```python
from build123d import *

# Parameters (mm, degrees)
IZIM1_R                     = 10
Y_KSEKLIK_EKSTR_ZYON1_DEPTH = 215
Y_KSEKLIK_EKSTR_ZYON2_DEPTH = 150


with BuildPart() as part:
    # Çizim1 → Yükseklik-Ekstrüzyon1 (new body)
    with BuildSketch(Plane.XY):
        Circle(IZIM1_R)
    extrude(amount=-Y_KSEKLIK_EKSTR_ZYON1_DEPTH)

    # Çizim2 → Yükseklik-Ekstrüzyon2 (add)
    with BuildSketch(Plane.XY.offset(-40)):
        with BuildLine():
            ThreePointArc((-9.797958971, -2), (-10, 0), (-9.797958971, 2))
            Line((-9.797958971, 2), (-11.832159566, 2))
            ThreePointArc((-11.832159566, 2), (-12, 0), (-11.832159566, -2))
            Line((-11.832159566, -2), (-9.797958971, -2))
        make_face()
        with BuildLine():
            Line((-1.1256228, 9.936446715), (-1.754225354, 11.871086446))
            ThreePointArc((-1.754225354, 11.871086446), (-3.708203932, 11.412678196), (-5.558451419, 10.635018469))
            Line((-5.558451419, 10.635018469), (-4.929848865, 8.700378737))
            ThreePointArc((-4.929848865, 8.700378737), (-3.090169944, 9.510565163), (-1.1256228, 9.936446715))
        make_face()
        with BuildLine():
            Line((8.396847665, 8.572802885), (6.751144813, 7.377129775))
            ThreePointArc((6.751144813, 7.377129775), (8.090169944, 5.877852523), (9.102285822, 4.141061797))
            Line((9.102285822, 4.141061797), (10.747988674, 5.336734907))
            ThreePointArc((10.747988674, 5.336734907), (9.708203932, 7.053423028), (8.396847665, 8.572802885))
        make_face()
        with BuildLine():
            Line((10.747988674, -5.336734907), (9.102285822, -4.141061797))
            ThreePointArc((9.102285822, -4.141061797), (8.090169944, -5.877852523), (6.751144813, -7.377129775))
            Line((6.751144813, -7.377129775), (8.396847665, -8.572802885))
            ThreePointArc((8.396847665, -8.572802885), (9.708203932, -7.053423028), (10.747988674, -5.336734907))
        make_face()
        with BuildLine():
            ThreePointArc((-1.1256228, -9.936446715), (-3.090169944, -9.510565163), (-4.929848865, -8.700378737))
            Line((-4.929848865, -8.700378737), (-5.558451419, -10.635018469))
            ThreePointArc((-5.558451419, -10.635018469), (-3.708203932, -11.412678196), (-1.754225354, -11.871086446))
            Line((-1.754225354, -11.871086446), (-1.1256228, -9.936446715))
        make_face()
    extrude(amount=-Y_KSEKLIK_EKSTR_ZYON2_DEPTH)


solid = part.part
```
Model file for the job. Use its own axes, mm. A direction names the side the tool comes from. Round coordinates to 2 decimals unless told otherwise and drop trailing zeros. Loops run counter-clockwise (first coordinate to the right, second up) from the corner with the lowest first, then second, coordinate; pieces in that order, holes last. Notation, with made-up numbers: M -19,16.25 L -10,16.25 A25 ccw -10,50.25 Z; hole C 32,12.5 d2. An arc over 180 degrees is marked long. Put each result on its own line as item: value. Start each with the question number.
Item 1: 3-axis set-ups, long thin cutter, end or side, ignore diameter. For faces 1 (the face through (9, 6, -190)), 2 (the face through (-3.735, -11.404, -113.95)), 3 (the face through (9, 6, -40)), 4 (the face through (9, -6, -190)), 5 (the face through (9, -6, -40)): which of +Z, -Z, +X, -X, +Y, -Y reach the whole face in a straight line?
Item 2: Cut at B-B (z = -91.5). List the corners of the cut face in (x, y), then the cut area to 3 significant figures.
Item 3: Drop flat-ended pins along their axis: P1, Ø1, axis at y = -7.5, z = -24.5, coming from the -X side; P2, Ø1, axis at x = -3, y = 10.5, coming from the -Z side; P3, Ø3, axis at y = 7, z = -192.5, coming from the +X side; P4, Ø1, axis at x = 6.5, y = -8.5, coming from the +Z side. Give the stop position or say it passes through.
Item 4: Drill centre lines: line 1 along Y through (x, z) = (-10.5, -57); line 2 along X through (y, z) = (6.75, -37); line 3 along Z through (x, y) = (8.25, -7). Where is each one in solid material? Low to high.
Item 5: Cut at C-C (x = 1). List the corners of the cut face in (y, z), then the cut area to 3 significant figures.
Item 6: Cut at A-A (y = 0). List the corners of the cut face in (x, z), then the cut area to 3 significant figures.
Answer block:
1. face 1: -Z, +X, +Y
1. face 2: +Z, -Z, -X, -Y
1. face 3: +Z, +X, +Y
1. face 4: -Z, +X, -Y
1. face 5: +Z, +X, -Y
2. outline: M -11.83,-2 L -9.8,-2 A10 ccw -4.93,-8.7 L -5.56,-10.64 A12 ccw -1.75,-11.87 L -1.13,-9.94 A10 ccw 6.75,-7.38 L 8.4,-8.57 A12 ccw 10.75,-5.34 L 9.1,-4.14 A10 ccw 9.1,4.14 L 10.75,5.34 A12 ccw 8.4,8.57 L 6.75,7.38 A10 ccw -1.13,9.94 L -1.75,11.87 A12 ccw -5.56,10.64 L -4.93,8.7 A10 ccw -9.8,2 L -11.83,2 A12 ccw Z
2. area: 354 mm2
3. P1: x = -7.14
3. P2: z = -190
3. P3: x = 8.35
3. P4: through
4. line 1: -2 to 2
4. line 2: -7.38 to 7.38
4. line 3: -190 to -40
5. outline: M -9.95,-215 L 9.95,-215 L 9.95,0 L -9.95,0 Z
5. area: 4,280 mm2
6. outline: M -12,-190 L -10,-190 L -10,-215 L 10,-215 L 10,0 L -10,0 L -10,-40 L -12,-40 Z
6. area: 4,600 mm2
